For this review, take the finished solid that the model builds, in its own axes (mm). A direction names the side the tool comes from. Round coordinates to 2 decimals unless told otherwise and drop trailing zeros. Order: outer loops, then holes, each group sorted by start corner. A loop starts at its lowest first (then second) coordinate and runs counter-clockwise, first axis right, second up.
Autodesk Inventor part; units mm, degrees
ref_plane "YZ Plane" through (0, 0, 0) normal (1, 0, 0) x (0, 1, 0)
ref_plane "XZ Plane" through (0, 0, 0) normal (0, 1, 0) x (-1, 0, 0)
ref_plane "XY Plane" through (0, 0, 0) normal (0, 0, 1) x (1, 0, 0)
sketch "Szkic1" plane through (0, 0, 0) normal (1, 0, 0) x (0, 1, 0)
  line L0 (0, 0) -> (41, 0)
  line L1 (41, 0) -> (41, -98)
  line L2 (41, -98) -> (0, -98)
  line L3 (0, -98) -> (0, 0)
  dimension "d0" = 98
  dimension "d1" = 41
extrude "Wyciągnięcie proste1" add sketch "Szkic1" along normal blind 15
sketch "Szkic2" plane through (15, 0, 0) normal (1, 0, 0) x (0, 0, -1)
  line L0 (4, 4) -> (94, 4)
  line L1 (94, 4) -> (94, 37)
  line L2 (94, 37) -> (4, 37)
  line L3 (4, 37) -> (4, 4)
  line L4 (49, 37) -> (49, 41) construction
  line L5 (98, 41) -> (0, 41)
  line L6 (94, 20.5) -> (98, 20.5) construction
  line L7 (98, 0) -> (98, 41)
  point P0 (0, 0)
  dimension "d4" = 90
  dimension "d5" = 33
extrude "Wyciągnięcie proste2" cut sketch "Szkic2" against normal blind 1.5
sketch "Szkic3" plane through (0, 0, 0) normal (-1, 0, 0) x (0, 0, 1)
  line L0 (-151.5, 53.7) -> (7.5, 53.7)
  line L1 (7.5, 53.7) -> (7.5, -6.3)
  line L2 (7.5, -6.3) -> (-151.5, -6.3)
  line L3 (-151.5, -6.3) -> (-151.5, 53.7)
  line L4 (-98, 41) -> (0, 41)
  line L5 (0, 41) -> (0, 0)
  line L6 (-98, 0) -> (0, 0)
  dimension "d8" = 159
  dimension "d9" = 60
  dimension "d10" = 7.5
  dimension "d11" = 6.3
extrude "Wyciągnięcie proste3" add sketch "Szkic3" along normal blind 2
sketch "Szkic4" plane through (0, 0, 0) normal (1, 0, 0) x (0, 0, -1)
  line L0 (110.5, 21) -> (144.5, 21) construction
  line L1 (127.5, 4) -> (127.5, 38) construction
  line L2 (98, 40.528) -> (98, -0.472) construction
  line L3 (98, 0) -> (98, 41)
  line L4 (0, 0) -> (98, 0)
  circle A0 centre (127.5, 38) radius 4
  circle A1 centre (110.5, 21) radius 4
  circle A2 centre (144.5, 21) radius 4
  circle A3 centre (127.5, 4) radius 4
  circle A4 centre (127.5, 21) radius 4
  dimension "d14" = 34
  dimension "d15" = 34
  dimension "d16" = 29.5
  dimension "d17" = 4
  dimension "d18" = 8
sketch "Szkic5" plane through (0, 0, 0) normal (1, 0, 0) x (0, 0, -1)
  line L0 (-4, -0.5) -> (149, -0.5) construction
  line L1 (149, -0.5) -> (149, 50.5) construction
  line L2 (149, 50.5) -> (-4, 50.5) construction
  line L3 (-4, 50.5) -> (-4, -0.5) construction
  line L4 (0, 41) -> (0, 0)
  line L5 (0, 0) -> (98, 0)
  dimension "d21" = 51
  dimension "d22" = 153
  dimension "d23" = 4
  dimension "d24" = 0.5
hole "Otwór1" at (0, -0.5, -149) at (0, 50.5, -149) at (0, 50.5, 4) at (0, -0.5, 4) direction (-1, 0, 0) diameter 3.5 end through all
extrude "Wyciągnięcie proste5" add sketch "Szkic4" along normal blind 17
properties part number "27_LCD"
Q1. Tool access review of faces 4 (the face through (7, 41, -48)), 5 (the face through (15, 3.7, -45.1)), 6 (the face through (7, 0, -50)), 7 (the face through (8.381, 3.824, -123.504)): name each direction out of +Z, -Z, +X, -X, +Y, -Y from which nothing blocks a thin tool from reaching the whole face with its end or side.
Q2. Take a section at A-A, the plane y = 50.5. State the section outline as (x, z) points, plus the area to 3 significant figures.
Q3. Clearance check with flat-ended pins moving along their axes: pin 1 (0.8 mm diameter, centred on x = 14, y = 22, fed in from +Z); pin 2 (1.5 mm diameter, centred on x = 5.5, z = -13.5, fed in from +Y); pin 3 (0.8 mm diameter, centred on x = 14.5, z = -61, fed in from -Y); pin 4 (4.5 mm diameter, centred on y = 50.5, z = 4, fed in from -X). State where each tip first meets the part, or that it passes through.
Q4. Wall thickness on line 1 (Y direction, x = -0.7, z = 4); line 2 (Z direction, x = -1.25, y = -0.5); line 3 (Z direction, x = 15.25, y = 23): over which ranges is each line inside the solid? List them lowest first.
Q5. Take a section at C-C, the plane z = -59. State the section outline as (x, y) points, plus the area to 4 significant figures.
Q6. Take a section at B-B, the plane x = 1.5. State the section outline as (y, z) points, plus the area to 3 significant figures.
Q7. Mouldability with a two-part tool opening along Z and no side actions: class faces 1 (the face through (8.38, 18.3, -124.55)), 2 (the face through (7, 20, 0)), 3 (the face through (-2, 24, -73)) as +Z half, -Z half, draft (parallel to the pull), parting line (faces both ways), or undercut.
Q8. Take a section at D-D, the plane y = 14. State the section outline as (x, z) points.
Working result:
1. face 4: +Z, +X, +Y
1. face 5: +Z, +X, +Y, -Y
1. face 6: +Z, -Z, +X, -Y
1. face 7: +X
2. outline: (-2, -151.5) - (0, -151.5) - (0, -150.75) - (-2, -150.75) - close; (-2, -147.25) - (0, -147.25) - (0, 2.25) - (-2, 2.25) - close; (-2, 5.75) - (0, 5.75) - (0, 7.5) - (-2, 7.5) - close
2. area: 304 mm2
3. pin 1: stops at z = 0
3. pin 2: stops at y = 41
3. pin 3: stops at y = 0
3. pin 4: stops at x = -2
4. line 1: y = -6.3 to -2.25, 1.25 to 48.75, 52.25 to 53.7
4. line 2: z = -151.5 to -150.75, -147.25 to 2.25, 5.75 to 7.5
4. line 3: z = -147.96 to -141.04, -130.96 to -124.04, -113.96 to -107.04
5. outline: (-2, -6.3) - (0, -6.3) - (0, 0) - (15, 0) - (15, 4) - (13.5, 4) - (13.5, 37) - (15, 37) - (15, 41) - (0, 41) - (0, 53.7) - (-2, 53.7) - close
5. area: 685.5 mm2
6. outline: circle Ø8 at (4, -127.5); (0, -98) - (41, -98) - (41, 0) - (0, 0) - close; circle Ø8 at (21, -144.5); circle Ø8 at (21, -127.5); circle Ø8 at (21, -110.5); circle Ø8 at (38, -127.5)
6. area: 4,270 mm2
7. face 1: undercut
7. face 2: +Z half
7. face 3: draft
8. outline: (-2, -151.5) - (0, -151.5) - (0, -98) - (15, -98) - (15, -94) - (13.5, -94) - (13.5, -4) - (15, -4) - (15, 0) - (0, 0) - (0, 7.5) - (-2, 7.5) - close
